Can you work these out from the drawing? Everything is in mm from the part's minimum corner. Give positions to 0.01 mm unless a question says otherwise; leave off trailing zeros. Write each loop counter-clockwise with the first axis right and the second up, starting at its lowest first coordinate (ties: lowest second). Pieces come first, ordered by that corner, then holes. Notation, with made-up numbers: (30, 24.25) -> (45, 24.25) arc R20 ccw to (45, 45.25) -> close; hole circle Ø3 at (5.25, 51.5). An arc over 180 degrees is marked (long way). Return JSON: item names as keys, results as strings.
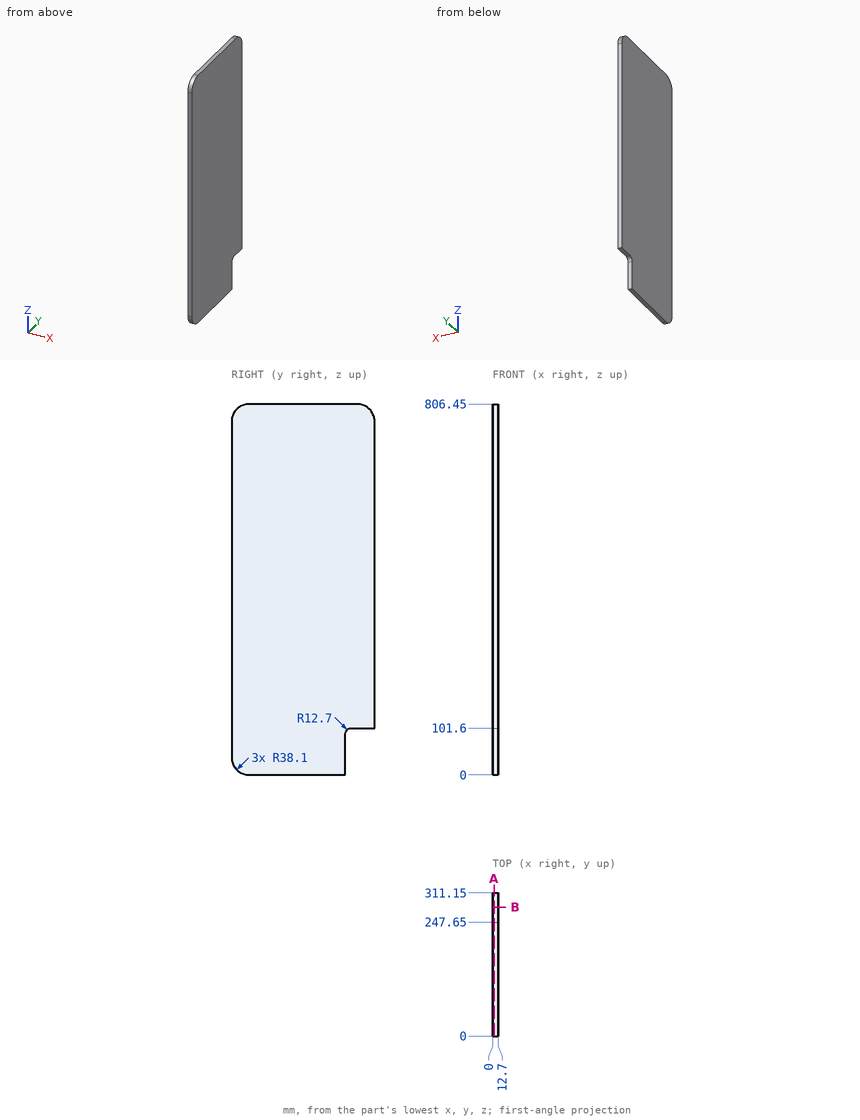
1. If I drill on line 1 (Z direction, x = 10.25, y = 35); line 2 (Y direction, x = 2.5, z = 60); line 3 (Z direction, x = 5.25, y = 278.5), over which ranges is the centre line in solid material (lowest first)? Write a range as [from, to].
Taken from the geometry:
{"line 1": "z = [0.13, 806.32]", "line 2": "y = [0, 247.65]", "line 3": "z = [101.6, 806.06]"}
2. For pin 1 Ø5 at (x, z) = (9.5, 719.5) entering from -Y; pin 2 Ø6 at (x, y) = (8, 33.5) entering from -Z; pin 3 Ø6.5 at (x, y) = (6, 289.5) entering from -Z, each with a flat end and sliding along its axis, tell me the tip position at first contact or that it passes through.
Taken from the geometry:
{"pin 1": "stops at y = 0", "pin 2": "stops at z = 0.03", "pin 3": "stops at z = 101.6"}
3. Suppose I cut it at A-A, the plane x = 3.25. List the corners of the cut face in (y, z) for me.
Taken from the geometry:
{"outline": "(0, 38.1) arc R38.1 ccw to (38.1, 0) -> (247.65, 0) -> (247.65, 88.9) arc R12.7 cw to (260.35, 101.6) -> (311.15, 101.6) -> (311.15, 768.35) arc R38.1 ccw to (273.05, 806.45) -> (38.1, 806.45) arc R38.1 ccw to (0, 768.35) -> close"}
4. Suppose I cut it at B-B, the plane y = 280. List the corners of the cut face in (x, z) for me, and give its area (3 significant figures).
Taken from the geometry:
{"outline": "(0, 101.6) -> (12.7, 101.6) -> (12.7, 805.81) -> (0, 805.81) -> close", "area": "8,940 mm²"}
